Could you check a few things on this drawing? It's one solid part, dimensions in mm from its lowest x, y, z. A direction names the side the tool comes from. Give positions to 0.01 mm unless a question says otherwise; leave off trailing zeros. Loops run counter-clockwise (first coordinate to the right, second up) from the corner with the lowest first, then second, coordinate; pieces in that order, holes last. Notation, with made-up numbers: (33, 12.5) - (85, 12.5) arc R24 ccw to (85, 26.5) - close; hole circle Ø3 at (41.5, 20.5). An arc over 180 degrees is marked (long way). Return JSON: item names as keys, results as strings. Group by question number.
(1) If we mould it in two halves opening along Y, with no side actions, what happens to the marked faces 1, 2 and 3? For each: released by +Y, released by -Y, zero draft, split by the parting line, or undercut.
(2) For P1, Ø3, axis at x = 2, z = 4.5, coming from the +Y side; P2, Ø1, axis at x = 3, z = 4, coming from the -Y side; P3, Ø3, axis at y = 4.5, z = 5.5, coming from the -X side, each with a flat end and sliding along its axis, tell me the tip position at first contact or that it passes through.
(3) On a 3-axis mill with a long thin cutter (end or side, diameter ignored), from which of +Z, -Z, +X, -X, +Y, -Y can I reach the whole of each face in a straight line? I mean the marked faces 4 and 5. Say none if no direction works.
(4) If we section it at C-C (z = 1.5): Please give me the cut outline in (x, y), then the cut area to 3 significant figures.
(5) If we section it at D-D (x = 0.4): Please give me the cut outline in (y, z), then the cut area to 3 significant figures.
(6) I need wall thicknesses on probe 1 along Y at (x, z) = (3, 5); probe 2 along Y at (x, z) = (3.95, 5.25); probe 3 along X at (y, z) = (3.55, 1). Which ranges of each line are inside material? Lowest first, please. Write a range as [from, to].
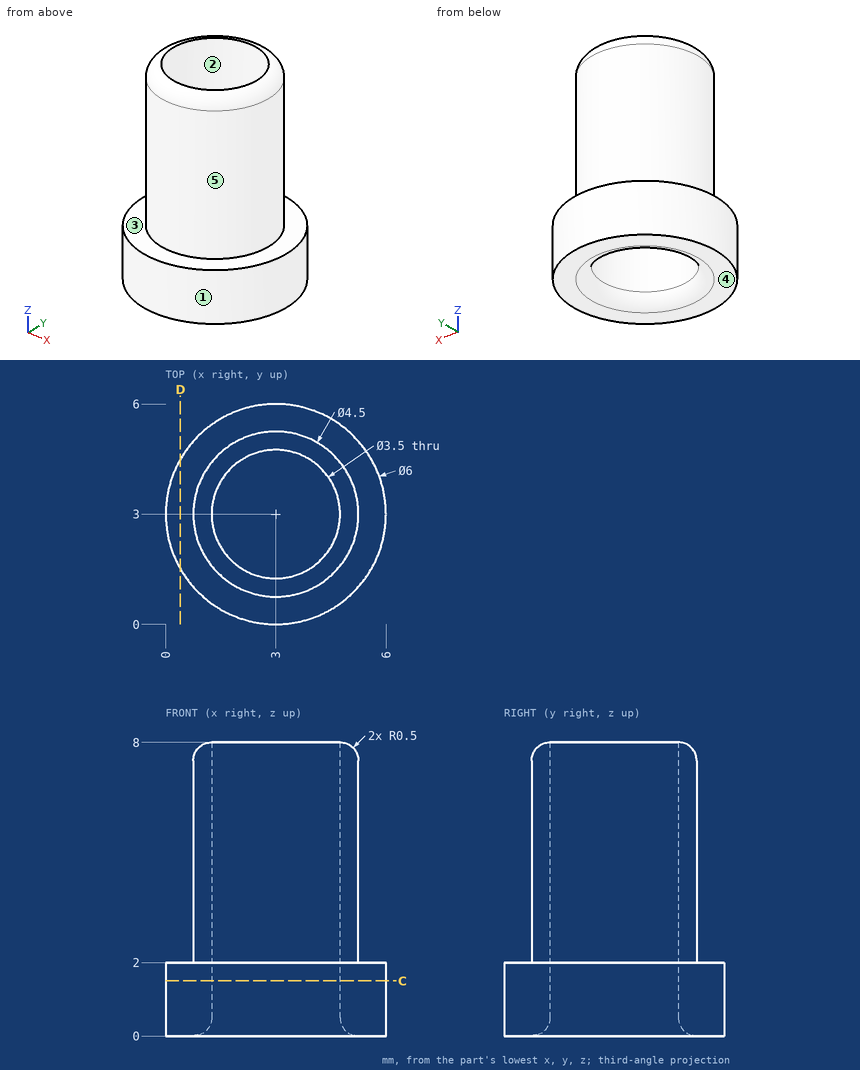
Values:
{
 "1": {"face 1": "split by the parting line", "face 2": "undercut", "face 3": "zero draft"},
 "2": {"P1": "y = 5.25", "P2": "y = 0.75", "P3": "x = 0.75"},
 "3": {"face 4": "-Z, +X, -X, +Y, -Y", "face 5": "+Z"},
 "4": {"outline": "circle Ø6 at (3, 3); hole circle Ø3.5 at (3, 3)", "area": "18.7 mm2"},
 "5": {"outline": "(1.5, 0) - (4.5, 0) - (4.5, 2) - (1.5, 2) - close", "area": "5.99 mm2"},
 "6": {"probe 1": "[0.75, 1.25], [4.75, 5.25]", "probe 2": "[0.96, 1.53], [4.47, 5.04]", "probe 3": "[0.05, 1.34], [4.66, 5.95]"}
}
